Read the model definition and answer for the solid it produces. Units are mm, in the model's axes. A direction names the side the tool comes from. Round coordinates to 2 decimals unless told otherwise and drop trailing zeros. Write each loop counter-clockwise with the first axis right and the second up, starting at its lowest first coordinate (ties: lowest second). Pieces come first, ordered by that corner, then holes. Notation, with made-up numbers: (25, 48) -> (55, 48) arc R18 ccw to (55, 53) -> close; hole circle Ø8 at (46, 37). An arc over 180 degrees is marked (long way). Return JSON: item names as keys, results as strings.
from build123d import *

# Parameters (mm, degrees)
BOSS_EXTRUDE1_DEPTH = 279.4
CUT_EXTRUDE1_REACH  = 281.4
SKETCH2_R           = 1.125613493


with BuildPart() as part:
    # Sketch1 → Boss-Extrude1 (new body)
    with BuildSketch(Plane(origin=(0, 0, 0), x_dir=(0, 0, -1), z_dir=(1, 0, 0))):
        with BuildLine():
            Line((15.612422091, 1.524), (25.4, 1.524))
            Line((25.4, 1.524), (25.4, 0))
            Line((25.4, 0), (0, 0))
            Line((0, 0), (0, 1.524))
            Line((0, 1.524), (9.787577909, 1.524))
            ThreePointArc((9.787577909, 1.524), (12.7, 4.436422091), (15.612422091, 1.524))
        make_face()
    extrude(amount=BOSS_EXTRUDE1_DEPTH)

    # Sketch2 → Cut-Extrude1 (cut, up to next)
    with BuildSketch(Plane(origin=(279.4, 0, 0), x_dir=(0, 0, -1), z_dir=(1, 0, 0)), mode=Mode.PRIVATE) as cut_extrude1_sk1:
        with Locations((12.7, 1.524)):
            Circle(SKETCH2_R)
    cut_extrude1_tool1 = extrude(cut_extrude1_sk1.sketch, amount=-CUT_EXTRUDE1_REACH, mode=Mode.PRIVATE) & part.part
    add(cut_extrude1_tool1.solids().sort_by_distance((279.4, 1.524, -12.7))[0], mode=Mode.SUBTRACT)


solid = part.part
Item 1: Section B-B (z = -3.5) is taken. Give the vertices of the cut face in (x, y), then the cut area to 3 significant figures.
Worked answers:
{"outline": "(0, 0) -> (279.4, 0) -> (279.4, 1.52) -> (0, 1.52) -> close", "area": "426 mm2"}
Item 2: Straight lines are drawn through the part: L1, parallel to Z at x = 32, y = 1.6; L2, parallel to Y at x = 131, z = -12.7; L3, parallel to Y at x = 188, z = -8. For each, find the intervals that lie inside material, in ascending order. Write a range as [from, to].
Worked answers:
{"L1": "z = [-15.61, -13.82], [-11.58, -9.79]", "L2": "y = [0, 0.4], [2.65, 4.44]", "L3": "y = [0, 1.52]"}
Item 3: Flat-ended cylindrical pins translate along their axes: pin 1 (11 mm diameter, centred on x = 153.5, z = -22, fed in from +Y); pin 2 (2 mm diameter, centred on x = 116, z = -14, fed in from +Y); pin 3 (1.5 mm diameter, centred on y = 4, z = -22, fed in from -X); pin 4 (2 mm diameter, centred on x = 187, y = 3.5, fed in from -Z). Find the tip coordinate at first contact, or state that the pin passes through.
Worked answers:
{"pin 1": "stops at y = 1.52", "pin 2": "stops at y = 4.42", "pin 3": "passes through", "pin 4": "stops at z = -15.44"}
Item 4: Section A-A (x = 215) is taken. Give the vertices of the cut face in (y, z), then the cut area to 3 significant figures.
Worked answers:
{"outline": "(0, -25.4) -> (1.52, -25.4) -> (1.52, -15.61) arc R2.91 ccw to (1.52, -9.79) -> (1.52, 0) -> (0, 0) -> close; hole circle Ø2.25 at (1.52, -12.7)", "area": "48.1 mm2"}
Item 5: A tool of negligible diameter and unlimited length cuts with its end or side. For faces 1 (the flat face through (138, 1.524, -5)), 2 (the flat face through (138, 1.524, -20)), 3 (the flat face through (138, 0, -13)), from which of +Z, -Z, +X, -X, +Y, -Y can it reach the whole face along a straight path? Write none if from no direction.
Worked answers:
{"face 1": "+Z, +X, -X, +Y", "face 2": "-Z, +X, -X, +Y", "face 3": "+Z, -Z, +X, -X, -Y"}
